from build123d import *

# Parameters (mm, degrees)
ESQUISSE1_W        = 203.2
ESQUISSE1_H        = 25.4
BOSS_EXTRU_1_DEPTH = 6
D_GAGEMENT_M31_D   = 3.2


with BuildPart() as part:
    # Esquisse1 → Boss.-Extru.1 (new body)
    with BuildSketch(Plane.XY):
        Rectangle(ESQUISSE1_W, ESQUISSE1_H)
    extrude(amount=BOSS_EXTRU_1_DEPTH)

    # Dégagement M31 (through all)
    with Locations(Plane(origin=(89.6, 0, 6), x_dir=(1, 0, 0), z_dir=(0, 0, 1))):
        with Locations((0, 0), (-32, 0), (-68.6, 0), (-110.6, 0), (-147.2, 0), (-179.2, 0)):
            Hole(D_GAGEMENT_M31_D / 2)


solid = part.part
Can you work these out from the model? Positions are in its coordinate system, mm. Round coordinates to 2 decimals unless told otherwise and drop trailing zeros. Use CSV: the item, a comma, the result in double quotes. Start each with the question number.
1) We'd pull the mould along X, two halves only. Please class faces 1 (the cylindrical face through (59.2, 0.07, 2.96)), 2 (the flat face through (-1, 0, 6)), 3 (the flat face through (101.6, 0, 3)): released by +X, released by -X, zero draft, split by the parting line, or undercut.
2) For pin 1 Ø1.5 at (x, y) = (69.5, 0.5) entering from -Z; pin 2 Ø3 at (x, y) = (-21, 0) entering from -Z, each with a flat end and sliding along its axis, tell me the tip position at first contact or that it passes through.
3) Please list where these lines run through material, in increasing order: probe 1 along Y at (x, z) = (-89.6, 2.9); probe 2 along Y at (x, z) = (90, 4.9). Write a range as [from, to].
Geometry results:
1,face 1,"undercut"
1,face 2,"zero draft"
1,face 3,"released by +X"
2,pin 1,"stops at z = 0"
2,pin 2,"passes through"
3,probe 1,"y = [-12.7, -1.6], [1.6, 12.7]"
3,probe 2,"y = [-12.7, -1.55], [1.55, 12.7]"
